Verification items for this drawing (mm, ordinates from the low corner). A direction names the side the tool comes from. Coordinates: 2 decimals unless noted, no trailing zeros. Write each loop counter-clockwise with the first axis right and the second up, starting at its lowest first coordinate (ties: lowest second). Pieces come first, ordered by that corner, then holes. Notation, with made-up numbers: (-16, -34.75) -> (-1, -34.75) arc R22 ccw to (-1, -26.75) -> close; hole circle Ø7 at (46.25, 25). An arc over 180 degrees is marked (long way). Use CSV: the item, a comma, the result in double quotes.
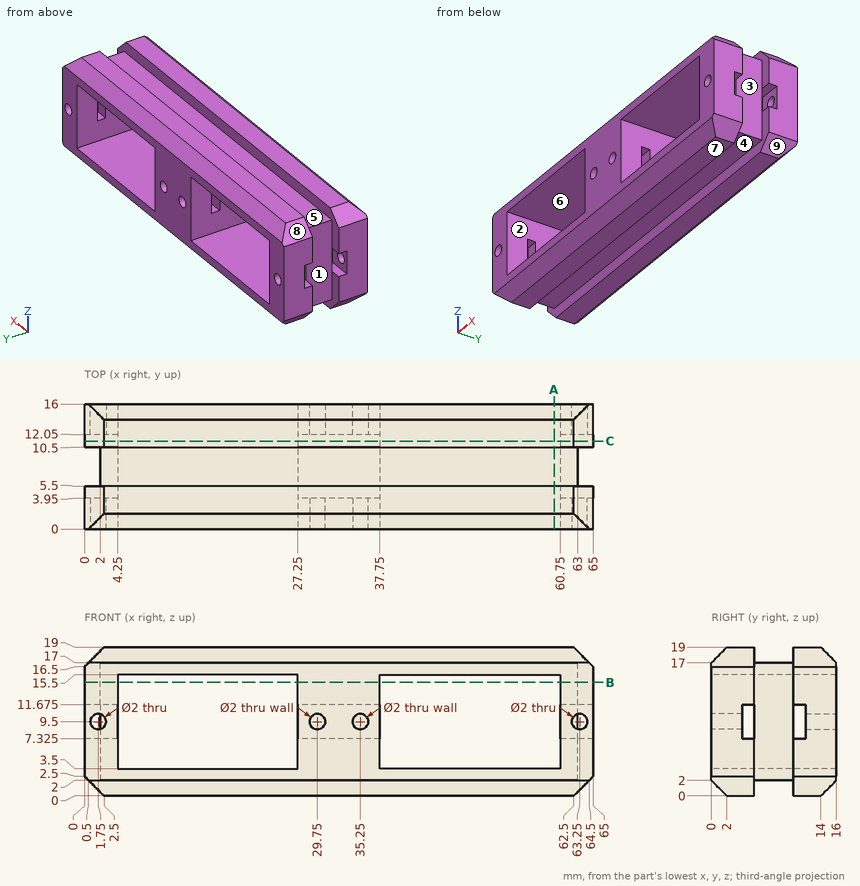
1) Cross-section at A-A (x = 60). Record the boundary of the cut face in (y, z), plus the area to 3 significant figures.
Return value:
outline,"(0, 2) -> (2, 0) -> (5.5, 0) -> (5.5, 2) -> (10.5, 2) -> (10.5, 0) -> (14, 0) -> (16, 2) -> (16, 3.5) -> (0, 3.5) -> close; (0, 15.5) -> (16, 15.5) -> (16, 17) -> (14, 19) -> (10.5, 19) -> (10.5, 17) -> (5.5, 17) -> (5.5, 19) -> (2, 19) -> (0, 17) -> close"
area,"84.0 mm2"
2) Cross-section at B-B (z = 14.5). Record the boundary of the cut face in (x, y), plus the area to 3 significant figures.
Return value:
outline,"(0, 0) -> (4.25, 0) -> (4.25, 16) -> (0, 16) -> (0, 10.5) -> (2, 10.5) -> (2, 5.5) -> (0, 5.5) -> close; (27.25, 0) -> (37.75, 0) -> (37.75, 16) -> (27.25, 16) -> close; (60.75, 0) -> (65, 0) -> (65, 5.5) -> (63, 5.5) -> (63, 10.5) -> (65, 10.5) -> (65, 16) -> (60.75, 16) -> close"
area,"284 mm2"
3) Mould release check, pull along X, two halves, no side actions. Record for the marked faces 6, 7, 8 and 9: released by +X, released by -X, zero draft, split by the parting line, or undercut.
Return value:
face 6,"undercut"
face 7,"zero draft"
face 8,"released by -X"
face 9,"released by +X"
4) Cross-section at C-C (y = 11.25). Record the boundary of the cut face in (x, z) (3 decimals), plus the area to 3 significant figures.
Return value:
outline,"(0, 2.5) -> (2.5, 0) -> (62.5, 0) -> (65, 2.5) -> (65, 7.325) -> (60.75, 7.325) -> (60.75, 3.5) -> (37.75, 3.5) -> (37.75, 7.325) -> (27.25, 7.325) -> (27.25, 3.5) -> (4.25, 3.5) -> (4.25, 7.325) -> (0, 7.325) -> close; (0, 11.675) -> (4.25, 11.675) -> (4.25, 15.5) -> (27.25, 15.5) -> (27.25, 11.675) -> (37.75, 11.675) -> (37.75, 15.5) -> (60.75, 15.5) -> (60.75, 11.675) -> (65, 11.675) -> (65, 16.5) -> (62.5, 19) -> (2.5, 19) -> (0, 16.5) -> close"
area,"588 mm2"
5) Gauge pin test, flat ends, axial feed: pin 1 (1.5 mm diameter, centred on x = 39, y = 8, fed in from -Z); pin 2 (1.7 mm diameter, centred on x = 64, y = 4.5, fed in from -Z); pin 3 (5.5 mm diameter, centred on y = 8, z = 9, fed in from +X). Record the tip position at first contact, or that the pin passes through.
Return value:
pin 1,"z = 2"
pin 2,"z = 0.65"
pin 3,"x = 63"
6) Scan lines: L1, parallel to X at y = 11, z = 6; L2, parallel to Z at x = 21.5, y = 12.75; L3, parallel to Z at x = 35.25, y = 2.3. Record each from-to range of solid material in increasing order.
Return value:
L1,"0 to 4.25, 27.25 to 37.75, 60.75 to 65"
L2,"0 to 3.5, 15.5 to 19"
L3,"0 to 8.5, 10.5 to 19"
7) Set-up check for the marked faces 1, 2, 3, 4 and 5: record each of +Z, -Z, +X, -X, +Y, -Y from which the full face is reachable in a straight line by a thin tool's end or side.
Return value:
face 1,"+Z, -Z, -X"
face 2,"+Y, -Y"
face 3,"+Z, -Z, +X"
face 4,"-Z, +X, -X"
face 5,"+Z, +X, -X"
